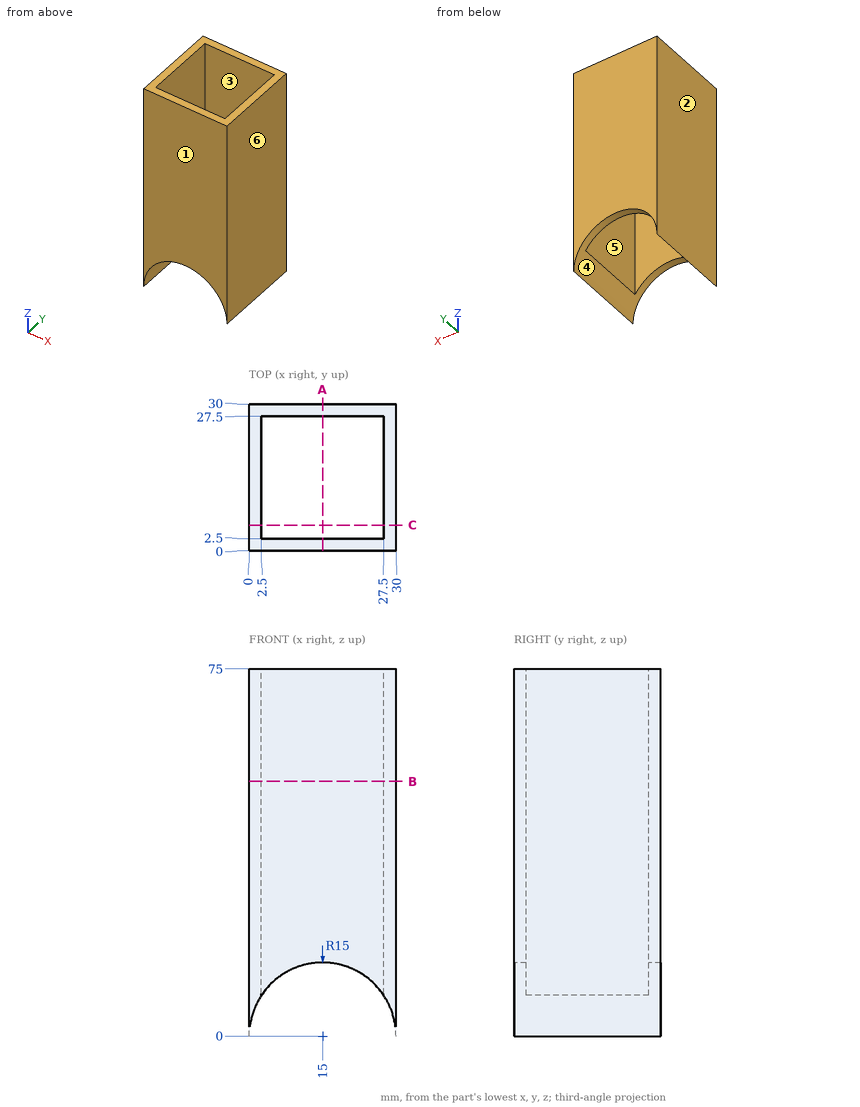
Study the drawing (mm; zero at the part's minimum x, y, z) and answer. A direction names the side the tool comes from. Give positions to 0.01 mm unless a question says otherwise; leave off trailing zeros. Write each loop counter-clockwise with the first axis right and the second up, starting at its lowest first coordinate (ties: lowest second). Pieces come first, ordered by that corner, then holes. Notation, with made-up numbers: (16.25, 73.5) -> (37.25, 73.5) arc R35 cw to (37.25, 109.5) -> close; hole circle Ø11 at (56.5, 51.5). An arc over 180 degrees is marked (long way). Write item = value, one per line. Start each with the question number.
1) Which of the six approach directions +Z, -Z, +X, -X, +Y, -Y give full straight-line access (tool end or side, diameter ignored) to the marked faces 5 and 6?
2) The part is cut by section C-C, the plane y = 5.25. Determine the outline of the cut face in (x, z).
3) The part is cut by section A-A, the plane x = 15. Determine the outline of the cut face in (y, z).
4) Determine the mould class of the marked faces 1, 2, 3 and 4 for opening direction X: +X half, -X half, draft (parallel to the pull), parting line (faces both ways), or undercut.
5) Straight lines are drawn through the part: line 1 along X through (y, z) = (22, 29); line 2 along X through (y, z) = (21, 6). For each, find the intervals that lie inside material, in ascending order.
6) The part is cut by section B-B, the plane z = 52. Determine the outline of the cut face in (x, y).
7) This flat-tipped pin is pushed along its axis until it touches: pin 1 (10 mm diameter, centred on x = 12.5, z = 32.5, fed in from -Y). Where does it stop, or does it pass through?
Solutions:
q1.face_5 = +Z, -Z
q1.face_6 = +Z, -Z, +X, +Y, -Y
q2.outline = (0, 0) arc R15 cw to (2.5, 8.29) -> (2.5, 75) -> (0, 75) -> close; (27.5, 8.29) arc R15 cw to (30, 0) -> (30, 75) -> (27.5, 75) -> close
q3.outline = (0, 15) -> (2.5, 15) -> (2.5, 75) -> (0, 75) -> close; (27.5, 15) -> (30, 15) -> (30, 75) -> (27.5, 75) -> close
q4.face_1 = draft
q4.face_2 = -X half
q4.face_3 = undercut
q4.face_4 = undercut
q5.line_1 = 0 to 2.5, 27.5 to 30
q5.line_2 = 0 to 1.25, 28.75 to 30
q6.outline = (0, 0) -> (30, 0) -> (30, 30) -> (0, 30) -> close; hole (2.5, 2.5) -> (27.5, 2.5) -> (27.5, 27.5) -> (2.5, 27.5) -> close
q7.pin_1 = 0
